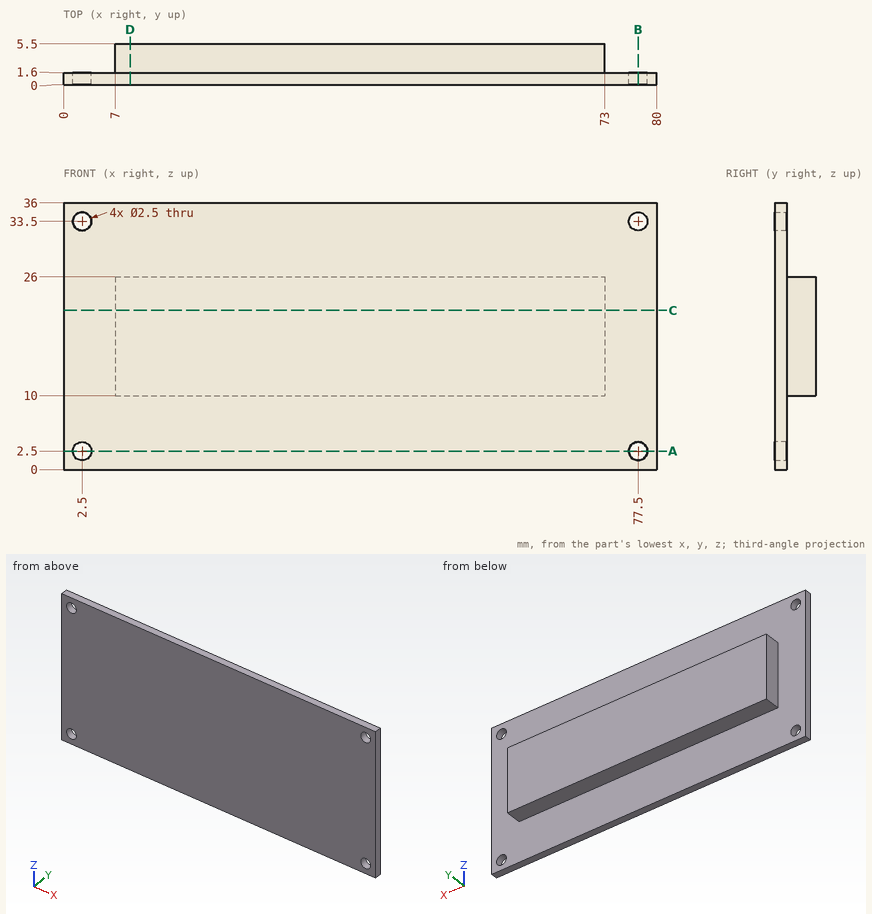
Geometry: see drawing. Coordinates: mm, zero at the bounding-box minimum. Coordinates: 2 decimals unless noted, no trailing zeros. Loops run counter-clockwise (first coordinate to the right, second up) from the corner with the lowest first, then second, coordinate; pieces in that order, holes last. Notation, with made-up numbers: M 63,85 L 86,85 A18 cw 86,102 Z; hole C 10,86 d3. An arc over 180 degrees is marked long. Put each result on its own line as item: value. Start each with the question number.
1) Contact query for flat-ended pins moving along their axis: pin 1 Ø1.2 at (y, z) = (2.5, 15) entering from +X; pin 2 Ø1.5 at (x, y) = (62, 2.5) entering from +Z; pin 3 Ø4 at (x, z) = (2.5, 2.5) entering from +Y. Output: stop coordinate, or through.
2) Cut plane A-A on z = 2.5. Return the cut outline in (x, y).
3) Cut plane D-D on x = 9. Return the cut outline in (y, z), then the cut area to 3 significant figures.
4) Ray query, L1, parallel to X at y = 1.25, z = 2.5; L2, parallel to X at y = 2.2, z = 12.5; L3, parallel to Y at x = 17.5, z = 8. Return the intervals inside material, ascending. Write a range as from..to.
5) Cut plane B-B on x = 77.5. Return the cut outline in (y, z).
6) Cut plane C-C on z = 21.5. Return the cut outline in (x, y), then the cut area to 3 significant figures.
The answers:
1. pin 1: stops at x = 73
1. pin 2: stops at z = 26
1. pin 3: stops at y = 1.6
2. outline: M 0,0 L 1.25,0 L 1.25,1.6 L 0,1.6 Z; M 3.75,0 L 76.25,0 L 76.25,1.6 L 3.75,1.6 Z; M 78.75,0 L 80,0 L 80,1.6 L 78.75,1.6 Z
3. outline: M 0,0 L 1.6,0 L 1.6,10 L 5.5,10 L 5.5,26 L 1.6,26 L 1.6,36 L 0,36 Z
3. area: 120 mm²
4. L1: x = 0..1.25, 3.75..76.25, 78.75..80
4. L2: x = 7..73
4. L3: y = 0..1.6
5. outline: M 0,0 L 1.6,0 L 1.6,1.25 L 0,1.25 Z; M 0,3.75 L 1.6,3.75 L 1.6,32.25 L 0,32.25 Z; M 0,34.75 L 1.6,34.75 L 1.6,36 L 0,36 Z
6. outline: M 0,0 L 80,0 L 80,1.6 L 73,1.6 L 73,5.5 L 7,5.5 L 7,1.6 L 0,1.6 Z
6. area: 385 mm²
